Check sheet for the modelled part. Datum: model origin and axes. Units: mm. Face numbers are marked on the shaded views. A direction names the side the tool comes from. Give positions to 0.01 mm unless a question says otherwise; leave off trailing zeros. Order: outer loops, then holes, each group sorted by start corner. A loop starts at its lowest first (then second) coordinate and runs counter-clockwise, first axis right, second up.
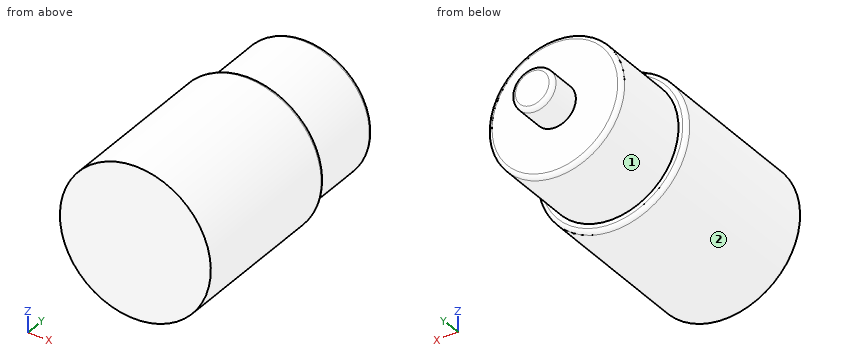
from build123d import *

# Parameters (mm, degrees)
SKETCH1_R           = 9
BOSS_EXTRUDE1_DEPTH = 20
SKETCH2_R           = 8
BOSS_EXTRUDE2_DEPTH = 10
SKETCH3_R           = 2.5
BOSS_EXTRUDE3_DEPTH = 4
FILLET1_R           = 0.5


with BuildPart() as part:
    # Sketch1 → Boss-Extrude1 (new body)
    with BuildSketch(Plane(origin=(0, 0, 0), x_dir=(1, 0, 0), z_dir=(0, 1, 0))):
        with Locations(Location((0, 0, 0), (0, 0, 270))):
            Circle(SKETCH1_R)
    extrude(amount=BOSS_EXTRUDE1_DEPTH)

    # Sketch2 → Boss-Extrude2 (add)
    with BuildSketch(Plane(origin=(0, 20, 0), x_dir=(1, 0, 0), z_dir=(0, 1, 0))):
        with Locations(Location((0, 0, 0), (0, 0, 270))):
            Circle(SKETCH2_R)
    extrude(amount=BOSS_EXTRUDE2_DEPTH)

    # Sketch3 → Boss-Extrude3 (add)
    with BuildSketch(Plane(origin=(0, 30, 0), x_dir=(1, 0, 0), z_dir=(0, 1, 0))):
        with Locations(Location((0, 0, 0), (0, 0, 270))):
            Circle(SKETCH3_R)
    extrude(amount=BOSS_EXTRUDE3_DEPTH)

    # Fillet1
    fillet1_edges = [part.edges().sort_by_distance(p)[0] for p in [
        (0, 34, -2.5),
        (0, 20, -9),
        (0, 30, -8),
    ]]
    fillet(fillet1_edges, radius=FILLET1_R)


solid = part.part
1) Depth check by flat-ended pin: pin 1 Ø1.5 at (x, y) = (4.5, 30.5) entering from -Z; pin 2 Ø2 at (x, y) = (-6, 21.5) entering from +Z (3 decimals); pin 3 Ø10 at (x, z) = (-5.5, -5.5) entering from +Y. Enter the tip coordinate at first touch or a pass-through.
Recorded:
pin 1: stops at z = -6.69
pin 2: stops at z = 6.245
pin 3: stops at y = 30
2) Section check C-C, the plane y = 27. Record the cut outline in (x, z).
Recorded:
outline: circle Ø16 at (0, 0)
3) Set-up check for the marked faces 1 and 2: record each of +Z, -Z, +X, -X, +Y, -Y from which the full face is reachable in a straight line by a thin tool's end or side.
Recorded:
face 1: +Y
face 2: +Y, -Y
4) Material ranges on L1, parallel to Z at x = -0.25, y = 21; L2, parallel to Y at x = 3.5, z = 2.5; L3, parallel to Y at x = 5.5, z = -6, recorded low to high.
Recorded:
L1: z = -8 to 8
L2: y = 0 to 30
L3: y = 0 to 20
5) Section check B-B, the plane z = 0. Record the cut outline in (x, y), then the cut area to 3 significant figures.
Recorded:
outline: (-9, 0) - (9, 0) - (9, 19.5) arc R0.5 ccw to (8.5, 20) - (8, 20) - (8, 29.5) arc R0.5 ccw to (7.5, 30) - (2.5, 30) - (2.5, 33.5) arc R0.5 ccw to (2, 34) - (-2, 34) arc R0.5 ccw to (-2.5, 33.5) - (-2.5, 30) - (-7.5, 30) arc R0.5 ccw to (-8, 29.5) - (-8, 20) - (-8.5, 20) arc R0.5 ccw to (-9, 19.5) - close
area: 540 mm2
6) Section check D-D, the plane y = 6. Record the cut outline in (x, z).
Recorded:
outline: circle Ø18 at (0, 0)
7) Section check A-A, the plane x = 0. Record the cut outline in (y, z), then the cut area to 3 significant figures.
Recorded:
outline: (0, -9) - (19.5, -9) arc R0.5 ccw to (20, -8.5) - (20, -8) - (29.5, -8) arc R0.5 ccw to (30, -7.5) - (30, -2.5) - (33.5, -2.5) arc R0.5 ccw to (34, -2) - (34, 2) arc R0.5 ccw to (33.5, 2.5) - (30, 2.5) - (30, 7.5) arc R0.5 ccw to (29.5, 8) - (20, 8) - (20, 8.5) arc R0.5 ccw to (19.5, 9) - (0, 9) - close
area: 540 mm2
